```python
from build123d import *

# Parameters (mm, degrees)
SKETCH_1_R          = 22.5
EXTRUDE_1_DEPTH     = 25
SKETCH_2_R          = 15.96
EXTRUDE_2_DEPTH     = 6
EXTRUDE_3_DEPTH     = 5.4
SKETCH_4_W          = 4.21
SKETCH_4_H          = 8.54
SKETCH_4_H_2        = 4.27
EXTRUDE_4_DEPTH     = 4.13
SKETCH_5_R          = 1.25
CUT_EXTRUDE_1_DEPTH = 3
SKETCH_6_R          = 3.6
CUT_EXTRUDE_2_DEPTH = 25


with BuildPart() as part:
    # 草图1 → 凸台-拉伸1 (new body)
    with BuildSketch(Plane(origin=(0, 0, 0), x_dir=(1, 0, 0), z_dir=(0, 1, 0))):
        with Locations(Location((0, 0, 0), (0, 0, 270))):
            Circle(SKETCH_1_R)
    extrude(amount=EXTRUDE_1_DEPTH)

    # 草图2 → 凸台-拉伸2 (add)
    with BuildSketch(Plane.XZ):
        with Locations(Location((0, 0, 0), (0, 0, 270))):
            Circle(SKETCH_2_R)
    extrude(amount=EXTRUDE_2_DEPTH)

    # 草图3 → 凸台-拉伸3 (add)
    with BuildSketch(Plane.XZ.offset(6)):
        with BuildLine():
            ThreePointArc((-6.4, 9), (-10.838477631, 10.838477631), (-9, 6.4))
            Line((-9, 6.4), (-9, 7.6))
            ThreePointArc((-9, 7.6), (-9.989949494, 9.989949494), (-7.6, 9))
            Line((-7.6, 9), (-6.4, 9))
        make_face()
        with BuildLine():
            Line((-9, 7.6), (-9, 6.4))
            ThreePointArc((-9, 6.4), (-7.161522369, 7.161522369), (-6.4, 9))
            Line((-6.4, 9), (-7.6, 9))
            ThreePointArc((-7.6, 9), (-8.010050506, 8.010050506), (-9, 7.6))
        make_face()
        with BuildLine():
            ThreePointArc((6.4, 9), (7.161522369, 7.161522369), (9, 6.4))
            Line((9, 6.4), (9, 7.6))
            ThreePointArc((9, 7.6), (8.010050506, 8.010050506), (7.6, 9))
            Line((7.6, 9), (6.4, 9))
        make_face()
        with BuildLine():
            Line((9, 7.6), (9, 6.4))
            ThreePointArc((9, 6.4), (10.838477631, 7.161522369), (11.6, 9))
            ThreePointArc((11.6, 9), (9, 11.6), (6.4, 9))
            Line((6.4, 9), (7.6, 9))
            ThreePointArc((7.6, 9), (9, 10.4), (10.4, 9))
            ThreePointArc((10.4, 9), (9.989949494, 8.010050506), (9, 7.6))
        make_face()
        with BuildLine():
            ThreePointArc((9, -6.4), (7.161522369, -7.161522369), (6.4, -9))
            Line((6.4, -9), (7.6, -9))
            ThreePointArc((7.6, -9), (8.010050506, -8.010050506), (9, -7.6))
            Line((9, -7.6), (9, -6.4))
        make_face()
        with BuildLine():
            Line((7.6, -9), (6.4, -9))
            ThreePointArc((6.4, -9), (9, -11.6), (11.6, -9))
            ThreePointArc((11.6, -9), (10.838477631, -7.161522369), (9, -6.4))
            Line((9, -6.4), (9, -7.6))
            ThreePointArc((9, -7.6), (9.989949494, -8.010050506), (10.4, -9))
            ThreePointArc((10.4, -9), (9, -10.4), (7.6, -9))
        make_face()
        with BuildLine():
            ThreePointArc((-9, -7.6), (-8.010050506, -8.010050506), (-7.6, -9))
            Line((-7.6, -9), (-6.4, -9))
            ThreePointArc((-6.4, -9), (-7.161522369, -7.161522369), (-9, -6.4))
            Line((-9, -6.4), (-9, -7.6))
        make_face()
        with BuildLine():
            Line((-6.4, -9), (-7.6, -9))
            ThreePointArc((-7.6, -9), (-9.989949494, -9.989949494), (-9, -7.6))
            Line((-9, -7.6), (-9, -6.4))
            ThreePointArc((-9, -6.4), (-10.838477631, -10.838477631), (-6.4, -9))
        make_face()
    extrude(amount=EXTRUDE_3_DEPTH)

    # 草图4 → 凸台-拉伸4 (add)
    with BuildSketch(Plane.XZ.offset(6)):
        with Locations((-11.985, 0)):
            Rectangle(SKETCH_4_W, SKETCH_4_H)
        with Locations((11.985, -2.135)):
            Rectangle(SKETCH_4_W, SKETCH_4_H_2)
        with Locations((11.985, 2.135)):
            Rectangle(SKETCH_4_W, SKETCH_4_H_2)
    extrude(amount=EXTRUDE_4_DEPTH)

    # 草图5 → 切除-拉伸1 (cut)
    with BuildSketch(Plane(origin=(0, 25, 0), x_dir=(1, 0, 0), z_dir=(0, 1, 0))):
        with Locations(Location((7.5, 0, 0), (0, 0, 270))):
            Circle(SKETCH_5_R)
        with Locations(Location((-7.5, 0, 0), (0, 0, 270))):
            Circle(SKETCH_5_R)
        with Locations(Location((0, 7.5, 0), (0, 0, 270))):
            Circle(SKETCH_5_R)
        with Locations(Location((0, -7.5, 0), (0, 0, 270))):
            Circle(SKETCH_5_R)
        with Locations(Location((6.717514421, 6.717514421, 0), (0, 0, 270))):
            Circle(SKETCH_5_R)
        with Locations(Location((-6.717514421, -6.717514421, 0), (0, 0, 270))):
            Circle(SKETCH_5_R)
        with Locations(Location((6.717514421, -6.717514421, 0), (0, 0, 270))):
            Circle(SKETCH_5_R)
        with Locations(Location((-6.717514421, 6.717514421, 0), (0, 0, 270))):
            Circle(SKETCH_5_R)
    extrude(amount=-CUT_EXTRUDE_1_DEPTH, mode=Mode.SUBTRACT)

    # 草图6 → 切除-拉伸2 (cut)
    with BuildSketch(Plane(origin=(0, 25, 0), x_dir=(1, 0, 0), z_dir=(0, 1, 0))):
        with Locations(Location((0, 0, 0), (0, 0, 270))):
            Circle(SKETCH_6_R)
    extrude(amount=-CUT_EXTRUDE_2_DEPTH, mode=Mode.SUBTRACT)


solid = part.part
```
CAD build for the part. Positions are in the model's coordinates, mm. A direction names the side the tool comes from. Give positions to 0.01 mm unless a question says otherwise; leave off trailing zeros. Order: outer loops, then holes, each group sorted by start corner. A loop starts at its lowest first (then second) coordinate and runs counter-clockwise, first axis right, second up. Notation, with made-up numbers: M 73.25,35 L 94.25,35 A21 cw 94.25,67 Z; hole C 13,70 d2. An arc over 180 degrees is marked long. Put each result on its own line as item: value. Start each with the question number.
(1) Mould opens along Z. For faces 1 (the flat face through (-14.09, -8, 0)), 2 (the cylindrical face through (15.824, -2.958, 2.078)), 3 (the flat face through (-9.88, -8, 0)) say: +Z half, -Z half, draft (parallel to the pull), parting line (faces both ways), or undercut.
(2) Saw through at D-D, the plane y = 14. Write the cut outline in (x, z).
(3) Flat gauge pins, fed straight in: pin 1 Ø3 at (x, z) = (0, 7.5) entering from -Y; pin 2 Ø8 at (x, z) = (-15, -4.5) entering from -Y; pin 3 Ø6 at (y, z) = (20.5, 16) entering from +X. Where does each tip first touch, or does it go through?
(4) Drill centre lines: line 1 along X through (y, z) = (23, 0); line 2 along X through (y, z) = (-7.95, -9); line 3 along X through (y, z) = (7, 0). Where is each one in solid material? Low to high.
(5) Saw through at C-C, the plane x = 11. Write the cut outline in (y, z), then the cut area to 3 significant figures.
(6) Saw through at A-A, the plane y = -7. Give the number of separate pieces and of enclosed holes in the cut face, then the cut area to 3 significant figures.
(7) Which spindle directions (+Z, -Z, +X, -X, +Y, -Y) get a long thin tool onto all of the face, cutting with end or side? Do faces 4 (the flat face through (10.1, -11.4, -10.1)), 5 (the flat face through (9, -6, 9)), 6 (the flat face through (-12, -8, 4.27)), 7 (the cylindrical face through (-6.34, 23.52, 7.91)). Say none if no direction does.
Check result:
1. face 1: draft
1. face 2: parting line
1. face 3: undercut
2. outline: C 0,0 d45; hole C 0,0 d7.2
3. pin 1: stops at y = -6
3. pin 2: stops at y = -10.13
3. pin 3: stops at x = 18.36
4. line 1: x = -22.5 to -8.75, -6.25 to -3.6, 3.6 to 6.25, 8.75 to 22.5
4. line 2: x = -11.6 to -10.4, -7.6 to -6.4, 6.4 to 7.6, 10.4 to 11.6
4. line 3: x = -22.5 to -3.6, 3.6 to 22.5
5. outline: M -11.4,-10.66 L -6,-10.66 L -6,-11.56 L 0,-11.56 L 0,-19.63 L 25,-19.63 L 25,19.63 L 0,19.63 L 0,11.56 L -6,11.56 L -6,10.66 L -11.4,10.66 L -11.4,7.34 L -6,7.34 L -6,4.27 L -10.13,4.27 L -10.13,-4.27 L -6,-4.27 L -6,-7.34 L -11.4,-7.34 Z
5. area: 1,190 mm2
6. separate pieces: 6
6. enclosed holes: 4
6. area: 132 mm2
7. face 4: +Z, -Z, +X, -X, -Y
7. face 5: -Y
7. face 6: +X, -X, -Y
7. face 7: +Y
